For this review, take the finished solid that the model builds, in its own axes (mm). Coordinates: 2 decimals unless noted, no trailing zeros. Write each loop counter-clockwise with the first axis right and the second up, starting at its lowest first coordinate (ties: lowest second). Pieces come first, ordered by that corner, then holes. Notation, with made-up numbers: M -28,60.25 L -21,60.25 A5 cw -21,64.25 Z; hole C -19.5,73.5 d11. An arc over 180 degrees is marked long. One line per question, with ' | ' between items.
from build123d import *

# Parameters (mm, degrees)
F0_W     = 1117.6
F0_H     = 260.35
F1_DEPTH = 19.05
F2_W     = 6.35
F2_H     = 6.35
F3_DEPTH = 1117.601
F4_W     = 6.35
F4_H     = 6.35
F5_DEPTH = 1117.601


with BuildPart() as f1:
    # F0 (on Front) → F1 (new body)
    with BuildSketch(Plane.XZ):
        with Locations((-41.18352, -372.617407)):
            Rectangle(F0_W, F0_H)
    extrude(amount=F1_DEPTH)

    # F2 (on face) → F3 (cut, through all)
    with BuildSketch(Plane.YZ.offset(517.61648)):
        with Locations((-9.525, -245.617407)):
            Rectangle(F2_W, F2_H)
    extrude(amount=-F3_DEPTH, mode=Mode.SUBTRACT)

    # F4 (on face) + F2 (on face) → F5 (cut, through all)
    with BuildSketch(Plane.YZ.offset(517.61648)):
        with Locations((-15.875, -499.617407)):
            Rectangle(F4_W, F4_H)
        with Locations((-3.175, -499.617407)):
            Rectangle(F4_W, F4_H)
    with BuildSketch(Plane.YZ.offset(517.61648)):
        with Locations((-9.525, -245.617407)):
            Rectangle(F2_W, F2_H)
    extrude(amount=-F5_DEPTH, mode=Mode.SUBTRACT)


solid = f1.part
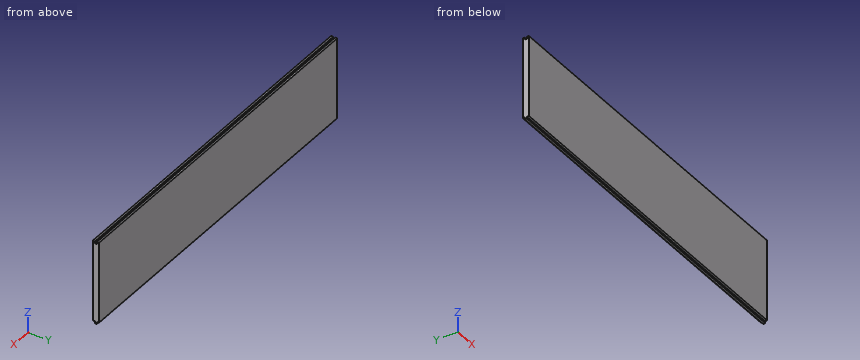
1. Take a section at A-A on x = 421.5. State the section outline as (y, z) points, plus the area to 3 significant figures.
Computed values:
outline: M -19.05,-496.44 L -12.7,-496.44 L -12.7,-502.79 L -6.35,-502.79 L -6.35,-496.44 L 0,-496.44 L 0,-242.44 L -6.35,-242.44 L -6.35,-248.79 L -12.7,-248.79 L -12.7,-242.44 L -19.05,-242.44 Z | area: 4,840 mm2
2. Clearance check with flat-ended pins moving along their axes: P1, Ø5, axis at x = -64.5, y = -16, coming from the -Z side; P2, Ø5, axis at x = -176.5, z = -500.5, coming from the -Y side; P3, Ø5, axis at x = -201.5, y = -10, coming from the +Z side. State where each tip first meets the part, or that it passes through.
Computed values:
P1: stops at z = -496.44 | P2: stops at y = -12.7 | P3: stops at z = -248.79
3. For line 1 along Z through (x, y) = (286, -11.25); line 2 along Z through (x, y) = (-189, -16), list the stretches that pass through material, from the lowest coordinate up.
Computed values:
line 1: z = -502.79 to -248.79 | line 2: z = -496.44 to -242.44
4. Take a section at B-B on y = -15.75. State the section outline as (x, z) points.
Computed values:
outline: M -599.98,-496.44 L 517.62,-496.44 L 517.62,-242.44 L -599.98,-242.44 Z
